```python
from build123d import *

# Parameters (mm, degrees)
SKETCH_1_R          = 1.5
SKETCH_1_R_2        = 13.5
EXTRUDE_1_DEPTH     = 5
SKETCH_2_W          = 45
SKETCH_2_H          = 6
EXTRUDE_2_DEPTH     = 45
CUT_EXTRUDE_1_REACH = 82.543
SKETCH_4_R          = 1.5
EXTRUDE_3_DEPTH     = 3
EXTRUDE_4_DEPTH     = 3
FILLET_1_R          = 1
CUT_EXTRUDE_2_DEPTH = 3
EXTRUDE_START       = 5
EXTRUDE_5_DEPTH     = 5
CUT_EXTRUDE_3_REACH = 85.14
SKETCH_9_R          = 7.5


with BuildPart() as part:
    # 草图1 → 凸台-拉伸1 (new body)
    with BuildSketch(Plane(origin=(0, 0, 0), x_dir=(1, 0, 0), z_dir=(0, 1, 0))):
        with BuildLine():
            ThreePointArc((0, 22.5), (6.590097423, 6.590097423), (22.5, 0))
            ThreePointArc((22.5, 0), (38.409902577, 6.590097423), (45, 22.5))
            Line((45, 22.5), (45, 47.5))
            Line((45, 47.5), (0, 47.5))
            Line((0, 47.5), (0, 22.5))
        make_face()
        with Locations(Location((10.125, 10.125, 0), (0, 0, 270))):
            Circle(SKETCH_1_R, mode=Mode.SUBTRACT)
        with Locations(Location((34.875, 10.125, 0), (0, 0, 270))):
            Circle(SKETCH_1_R, mode=Mode.SUBTRACT)
        with Locations(Location((22.5, 22.5, 0), (0, 0, 270))):
            Circle(SKETCH_1_R_2, mode=Mode.SUBTRACT)
        with Locations(Location((10.125, 34.875, 0), (0, 0, 270))):
            Circle(SKETCH_1_R, mode=Mode.SUBTRACT)
        with Locations(Location((34.875, 34.875, 0), (0, 0, 270))):
            Circle(SKETCH_1_R, mode=Mode.SUBTRACT)
    extrude(amount=EXTRUDE_1_DEPTH)

    # 草图2 → 凸台-拉伸2 (add)
    with BuildSketch(Plane(origin=(0, 5, 0), x_dir=(1, 0, 0), z_dir=(0, 1, 0))):
        with Locations((22.5, 50.5)):
            Rectangle(SKETCH_2_W, SKETCH_2_H)
    extrude(amount=-EXTRUDE_2_DEPTH)

    # 草图4 → 切除-拉伸1 (cut, up to next)
    with BuildSketch(Plane(origin=(0, 0, -53.5), x_dir=(-1, 0, 0), z_dir=(0, 0, -1)), mode=Mode.PRIVATE) as cut_extrude_1_sk1:
        with Locations((-9.5, -4.5)):
            Circle(SKETCH_4_R)
    cut_extrude_1_tool1 = extrude(cut_extrude_1_sk1.sketch, amount=-CUT_EXTRUDE_1_REACH, mode=Mode.PRIVATE) & part.part
    # 草图4 → 切除-拉伸1 (cut, up to next)
    with BuildSketch(Plane(origin=(0, 0, -53.5), x_dir=(-1, 0, 0), z_dir=(0, 0, -1)), mode=Mode.PRIVATE) as cut_extrude_1_sk2:
        with Locations((-9.5, -30.5)):
            Circle(SKETCH_4_R)
    cut_extrude_1_tool2 = extrude(cut_extrude_1_sk2.sketch, amount=-CUT_EXTRUDE_1_REACH, mode=Mode.PRIVATE) & part.part
    # 草图4 → 切除-拉伸1 (cut, up to next)
    with BuildSketch(Plane(origin=(0, 0, -53.5), x_dir=(-1, 0, 0), z_dir=(0, 0, -1)), mode=Mode.PRIVATE) as cut_extrude_1_sk3:
        with Locations((-35.5, -30.5)):
            Circle(SKETCH_4_R)
    cut_extrude_1_tool3 = extrude(cut_extrude_1_sk3.sketch, amount=-CUT_EXTRUDE_1_REACH, mode=Mode.PRIVATE) & part.part
    # 草图4 → 切除-拉伸1 (cut, up to next)
    with BuildSketch(Plane(origin=(0, 0, -53.5), x_dir=(-1, 0, 0), z_dir=(0, 0, -1)), mode=Mode.PRIVATE) as cut_extrude_1_sk4:
        with Locations((-35.5, -4.5)):
            Circle(SKETCH_4_R)
    cut_extrude_1_tool4 = extrude(cut_extrude_1_sk4.sketch, amount=-CUT_EXTRUDE_1_REACH, mode=Mode.PRIVATE) & part.part
    add(cut_extrude_1_tool1.solids().sort_by_distance((9.5, -4.5, -53.5))[0], mode=Mode.SUBTRACT)
    add(cut_extrude_1_tool2.solids().sort_by_distance((9.5, -30.5, -53.5))[0], mode=Mode.SUBTRACT)
    add(cut_extrude_1_tool3.solids().sort_by_distance((35.5, -30.5, -53.5))[0], mode=Mode.SUBTRACT)
    add(cut_extrude_1_tool4.solids().sort_by_distance((35.5, -4.5, -53.5))[0], mode=Mode.SUBTRACT)

    # 草图5 → 凸台-拉伸3 (add)
    with BuildSketch(Plane.ZY):
        Polygon((-47.5, 0), (-35, 0), (-47.5, -12.5), align=None)
    extrude(amount=-EXTRUDE_3_DEPTH)

    # 草图6 → 凸台-拉伸4 (add)
    with BuildSketch(Plane(origin=(45, 0, 0), x_dir=(0, 0, -1), z_dir=(1, 0, 0))):
        Polygon((35, 0), (47.5, 0), (47.5, -12.5), align=None)
    extrude(amount=-EXTRUDE_4_DEPTH)

    # 圆角1
    fillet_1_edges = [part.edges().sort_by_distance(p)[0] for p in [
        (22.5, 0, -47.5),
    ]]
    fillet(fillet_1_edges, radius=FILLET_1_R)

    # 草图7 → 切除-拉伸2 (cut)
    with BuildSketch(Plane.XY.offset(-47.5)):
        Polygon((11.08771324, -33.25), (7.91228676, -33.25), (6.324573519, -30.5), (7.91228676, -27.75), (11.08771324, -27.75), (12.675426481, -30.5), align=None)
        Polygon((37.08771324, -33.25), (38.675426481, -30.5), (37.08771324, -27.75), (33.91228676, -27.75), (32.324573519, -30.5), (33.91228676, -33.25), align=None)
        Polygon((33.91228676, -1.75), (37.08771324, -1.75), (38.675426481, -4.5), (37.08771324, -7.25), (33.91228676, -7.25), (32.324573519, -4.5), align=None)
        Polygon((7.91228676, -1.75), (6.324573519, -4.5), (7.91228676, -7.25), (11.08771324, -7.25), (12.675426481, -4.5), (11.08771324, -1.75), align=None)
    extrude(amount=-CUT_EXTRUDE_2_DEPTH, mode=Mode.SUBTRACT)

    # 草图8 → 凸台-拉伸5 (add)
    with BuildSketch(Plane(origin=(0, -40, 0), x_dir=(-1, 0, 0), z_dir=(0, -1, 0)).offset(EXTRUDE_START)):
        with BuildLine():
            Line((-45, 53.5), (-45, 22.5))
            ThreePointArc((-45, 22.5), (-22.5, 0), (0, 22.5))
            Line((0, 22.5), (0, 53.5))
            Line((0, 53.5), (-45, 53.5))
        make_face()
    extrude(amount=-EXTRUDE_5_DEPTH)

    # 草图9 → 切除-拉伸3 (cut, up to next)
    with BuildSketch(Plane(origin=(0, -40, 0), x_dir=(-1, 0, 0), z_dir=(0, -1, 0)), mode=Mode.PRIVATE) as cut_extrude_3_sk1:
        with Locations(Location((-22.5, 22.5, 0), (0, 0, 90))):
            Circle(SKETCH_9_R)
    cut_extrude_3_tool1 = extrude(cut_extrude_3_sk1.sketch, amount=CUT_EXTRUDE_3_REACH, mode=Mode.PRIVATE) & part.part
    add(cut_extrude_3_tool1.solids().sort_by_distance((22.5, -40, -22.5))[0], mode=Mode.SUBTRACT)


solid = part.part
```
Here's how the part is built. I have some questions about the finished solid (model axes, mm). A direction names the side the tool comes from. Round coordinates to 2 decimals unless told otherwise and drop trailing zeros. Order: outer loops, then holes, each group sorted by start corner. A loop starts at its lowest first (then second) coordinate and runs counter-clockwise, first axis right, second up. Notation, with made-up numbers: M 63.5,12 L 85.5,12 A17 cw 85.5,24 Z; hole C -36.75,-38.75 d8. An arc over 180 degrees is marked long. Answer in a Markdown table with one row per item.
Item 1: Imagine slicing it at C-C, the plane y = 1.5. Write out the boundary of the cut face in (x, z) (3 decimals), and give its area (3 significant figures).
A:
| item | result |
|---|---|
| outline | M 0,-53.5 L 45,-53.5 L 45,-22.5 A22.5 ccw 0,-22.5 Z; hole C 10.125,-34.875 d3; hole C 10.125,-10.125 d3; hole C 22.5,-22.5 d27; hole C 34.875,-34.875 d3; hole C 34.875,-10.125 d3 |
| area | 1,590 mm2 |
Item 2: If I drill on L1, parallel to Y at x = 35.5, z = -51.6; L2, parallel to Z at x = 22.5, y = -43.05; L3, parallel to Y at x = 36, z = -41, over which ranges is the centre line in solid material (lowest first)? Write a range as from..to.
A:
| item | result |
|---|---|
| L1 | y = -45..-32, -29..-6, -3..5 |
| L2 | z = -53.5..-30, -15..0 |
| L3 | y = -45..-40, 0..5 |
Item 3: Imagine slicing it at A-A, the plane z = -45. Write out the boundary of the cut face in (x, y), and give its area (3 significant figures).
A:
| item | result |
|---|---|
| outline | M 0,-45 L 45,-45 L 45,-40 L 0,-40 Z; M 0,-10 L 3,-10 L 3,0 L 42,0 L 42,-10 L 45,-10 L 45,5 L 0,5 Z |
| area | 510 mm2 |
Item 4: Thinking about a two-plate mould opening in Z: for faces 1 (the face through (22, -20, -53.5)), 2 (the face through (37.87, -3.106, -48.979)), 3 (the face through (27.6, -42.5, -17)), 4 (the face through (9.212, 2.465, -11.315)), which applies, +Z half, -Z half, draft (parallel to the pull), parting line (faces both ways), or undercut?
A:
| item | result |
|---|---|
| face 1 | -Z half |
| face 2 | draft |
| face 3 | undercut |
| face 4 | undercut |
Item 5: Imagine slicing it at B-B, the plane x = 19.5. Write out the boundary of the cut face in (y, z).
A:
| item | result |
|---|---|
| outline | M -45,-53.5 L 5,-53.5 L 5,-35.66 L 0,-35.66 L 0,-46.5 A1 cw -1,-47.5 L -40,-47.5 L -40,-29.37 L -45,-29.37 Z; M -45,-15.63 L -40,-15.63 L -40,-0.2 L -45,-0.2 Z; M 0,-9.34 L 5,-9.34 L 5,-0.2 L 0,-0.2 Z |
Item 6: I'm going to push flat-ended pins straight in: pin 1 (8 mm diameter, centred on y = -37, z = -40.5, fed in from +X); pin 2 (3 mm diameter, centred on x = 10.5, y = -5.5, fed in from +Z); pin 3 (3 mm diameter, centred on x = 10, y = -29.5, fed in from +Z); pin 4 (1.8 mm diameter, centred on x = 34.875, z = -10.125, fed in from +Y). Where does each tip first touch, or does it pass through?
A:
| item | result |
|---|---|
| pin 1 | stops at x = 45 |
| pin 2 | stops at z = -47.5 |
| pin 3 | stops at z = -50.5 |
| pin 4 | stops at y = -40 |
Item 7: For faces 5 (the face through (37.89, -5.86, -48.98)), 6 (the face through (0, -20, -48)), which set-ups out of +Z, -Z, +X, -X, +Y, -Y let a thin tool reach every point of the face, with its end or its side?
A:
| item | result |
|---|---|
| face 5 | +Z |
| face 6 | +Z, -Z, -X, +Y, -Y |
Item 8: Imagine slicing it at D-D, the plane z = -21.5. Write out the boundary of the cut face in (x, y), and give its area (3 significant figures).
A:
| item | result |
|---|---|
| outline | M 0.02,-45 L 15.07,-45 L 15.07,-40 L 0.02,-40 Z; M 0.02,0 L 9.04,0 L 9.04,5 L 0.02,5 Z; M 29.93,-45 L 44.98,-45 L 44.98,-40 L 29.93,-40 Z; M 35.96,0 L 44.98,0 L 44.98,5 L 35.96,5 Z |
| area | 241 mm2 |
